from build123d import *

# Parameters (mm, degrees)
BOSS_EXTRU_1_DEPTH      = 10
BOSS_EXTRU_2_DEPTH      = 10
BOSS_EXTRU_2_DEPTH_BACK = 20
ESQUISSE2_W             = 69
ESQUISSE2_H             = 10
ESQUISSE3_W             = 50
ESQUISSE3_H             = 5
BOSS_EXTRU_3_DEPTH      = 15
CHANFREIN1_SIZE         = 5
ESQUISSE4_R             = 2.1
ENL_V_MAT_EXTRU_1_DEPTH = 15
ESQUISSE5_W             = 30
ESQUISSE5_H             = 5
BOSS_EXTRU_4_DEPTH      = 5
ESQUISSE6_W             = 50
ESQUISSE6_H             = 5
BOSS_EXTRU_5_DEPTH      = 15
CHANFREIN2_SIZE         = 5
ESQUISSE7_R             = 2.1
ENL_V_MAT_EXTRU_2_DEPTH = 15
ESQUISSE8_R             = 6
ENL_V_MAT_EXTRU_3_DEPTH = 20
CONG_1_R                = 5


with BuildPart() as part:
    # Esquisse1 → Boss.-Extru.1 (new body)
    with BuildSketch(Plane.XY):
        Polygon((0, 0), (0, 81), (-69, 81), (-69, 66), (-64, 66), (-64, 71), (-50, 71), (-50, 0), align=None)
    extrude(amount=BOSS_EXTRU_1_DEPTH)

    # Esquisse2 → Boss.-Extru.2 (add, two sides: drawn at the far end of the back side and taken through both)
    with BuildSketch(Plane.XY.offset(10).offset(-BOSS_EXTRU_2_DEPTH_BACK)):
        with Locations((-34.5, 76)):
            Rectangle(ESQUISSE2_W, ESQUISSE2_H)
    extrude(amount=BOSS_EXTRU_2_DEPTH + BOSS_EXTRU_2_DEPTH_BACK)

    # Esquisse3 → Boss.-Extru.3 (add)
    with BuildSketch(Plane(origin=(0, 0, 0), x_dir=(-1, 0, 0), z_dir=(0, 0, -1))):
        with Locations((25, 2.5)):
            Rectangle(ESQUISSE3_W, ESQUISSE3_H)
    extrude(amount=BOSS_EXTRU_3_DEPTH)

    # Chanfrein1
    chanfrein1_edges = [part.edges().sort_by_distance(p)[0] for p in [
        (-25, 5, 0),
    ]]
    chamfer(chanfrein1_edges, length=CHANFREIN1_SIZE)

    # Esquisse4 → Enlèv. mat.-Extru.1 (cut)
    with BuildSketch(Plane(origin=(0, 5, 0), x_dir=(1, 0, 0), z_dir=(0, 1, 0))):
        with Locations(Location((-40, 10, 0), (0, 0, 180))):
            Circle(ESQUISSE4_R)
        with Locations(Location((-10, 10, 0), (0, 0, 180))):
            Circle(ESQUISSE4_R)
    extrude(amount=-ENL_V_MAT_EXTRU_1_DEPTH, mode=Mode.SUBTRACT)

    # Esquisse5 → Boss.-Extru.4 (add)
    with BuildSketch(Plane.ZY.offset(69)):
        with Locations((5, 68.5)):
            Rectangle(ESQUISSE5_W, ESQUISSE5_H)
    extrude(amount=-BOSS_EXTRU_4_DEPTH)

    # Esquisse6 → Boss.-Extru.5 (add)
    with BuildSketch(Plane.XY.offset(10)):
        with Locations((-25, 13.5)):
            Rectangle(ESQUISSE6_W, ESQUISSE6_H)
    extrude(amount=BOSS_EXTRU_5_DEPTH)

    # Chanfrein2
    chanfrein2_edges = [part.edges().sort_by_distance(p)[0] for p in [
        (-25, 11, 10),
    ]]
    chamfer(chanfrein2_edges, length=CHANFREIN2_SIZE)

    # Esquisse7 → Enlèv. mat.-Extru.2 (cut)
    with BuildSketch(Plane.XZ.offset(-11)):
        with Locations((-10, 20)):
            Circle(ESQUISSE7_R)
        with Locations((-40, 20)):
            Circle(ESQUISSE7_R)
    extrude(amount=-ENL_V_MAT_EXTRU_2_DEPTH, mode=Mode.SUBTRACT)

    # Esquisse8 → Enlèv. mat.-Extru.3 (cut)
    with BuildSketch(Plane(origin=(0, 81, 0), x_dir=(1, 0, 0), z_dir=(0, 1, 0))):
        with Locations(Location((-35, 0, 0), (0, 0, 270))):
            Circle(ESQUISSE8_R)
    extrude(amount=-ENL_V_MAT_EXTRU_3_DEPTH, mode=Mode.SUBTRACT)

    # Congé1
    # the kernel refuses this fillet: 5 mm, written as the material it adds along each edge
    with BuildSketch(Plane(origin=(0, 10, 0), x_dir=(0, -0.7071067811865476, -0.7071067811865476), z_dir=(-1, 0, 0)), Plane(origin=(0, 5, -5), x_dir=(0, 0, -1), z_dir=(-1, 0, 0))) as cong_1_piece_1:
        with BuildLine():
            CenterArc((CONG_1_R * 0.414213562373, -CONG_1_R), CONG_1_R, 90, 45)
            Line((-CONG_1_R * 0.292893218813, -CONG_1_R * 0.292893218813), (0, 0))
            Line((0, 0), (CONG_1_R * 0.414213562373, 0))
        make_face()
    extrude(amount=50)
    # the kernel refuses this fillet: 5 mm, written as the material it takes off along each edge
    with BuildSketch(Plane(origin=(-81.5, 81, 20), x_dir=(0, -1, 0), z_dir=(1, 0, 0))) as cong_1_2_piece_1:
        with BuildLine():
            CenterArc((CONG_1_R, CONG_1_R), CONG_1_R, 180, 90)
            Line((0, CONG_1_R), (0, 0))
            Line((0, 0), (CONG_1_R, 0))
        make_face()
    extrude(amount=94, mode=Mode.SUBTRACT)
    with BuildSketch(Plane(origin=(12.5, 71, 20), x_dir=(0, 0, -1), z_dir=(-1, 0, 0))) as cong_1_2_piece_2:
        with BuildLine():
            CenterArc((CONG_1_R, -CONG_1_R), CONG_1_R, 90, 90)
            Line((0, -CONG_1_R), (0, 0))
            Line((0, 0), (CONG_1_R, 0))
        make_face()
    extrude(amount=76.5, mode=Mode.SUBTRACT)
    with BuildSketch(Plane(origin=(0, 71, -2.5), x_dir=(0, 1, 0), z_dir=(0, 0, 1))) as cong_1_2_piece_3_section:
        with BuildLine():
            CenterArc((CONG_1_R, CONG_1_R), CONG_1_R, 180, 90)
            Line((0, CONG_1_R), (0, 0))
            Line((0, 0), (CONG_1_R, 0))
        make_face()
    cong_1_2_piece_3 = extrude(amount=35, mode=Mode.PRIVATE)
    cong_1_2_piece_3 = split(cong_1_2_piece_3, bisect_by=Plane(origin=(-1.116839695, 72.116839695, 0), z_dir=(0, 0, -1)), keep=Keep.TOP, mode=Mode.PRIVATE)
    add(cong_1_2_piece_3, mode=Mode.SUBTRACT)
    with BuildSketch(Plane(origin=(0, 71, 10), x_dir=(0, 1, 0), z_dir=(0, 0, 1)), Plane(origin=(0, 71, -22.5), x_dir=(0, 1, 0), z_dir=(0, 0, 1))) as cong_1_2_piece_4:
        with BuildLine():
            CenterArc((CONG_1_R, CONG_1_R), CONG_1_R, 180, 90)
            Line((0, CONG_1_R), (0, 0))
            Line((0, 0), (CONG_1_R, 0))
        make_face()
    extrude(amount=22.5, mode=Mode.SUBTRACT)
    with BuildSketch(Plane(origin=(0, 71, -22.5), x_dir=(0, 1, 0), z_dir=(0, 0, 1))) as cong_1_2_piece_5_section:
        with BuildLine():
            CenterArc((CONG_1_R, CONG_1_R), CONG_1_R, 180, 90)
            Line((0, CONG_1_R), (0, 0))
            Line((0, 0), (CONG_1_R, 0))
        make_face()
    cong_1_2_piece_5 = extrude(amount=35, mode=Mode.PRIVATE)
    cong_1_2_piece_5 = split(cong_1_2_piece_5, bisect_by=Plane(origin=(-1.116839695, 72.116839695, 10), z_dir=(0, 0, 1)), keep=Keep.TOP, mode=Mode.PRIVATE)
    add(cong_1_2_piece_5, mode=Mode.SUBTRACT)
    with BuildSketch(Plane(origin=(0, 81, -22.5), x_dir=(0, -1, 0), z_dir=(0, 0, 1)), Plane(origin=(-69, 81, -22.5), x_dir=(1, 0, 0), z_dir=(0, 0, 1))) as cong_1_2_piece_6:
        with BuildLine():
            CenterArc((CONG_1_R, -CONG_1_R), CONG_1_R, 90, 90)
            Line((0, -CONG_1_R), (0, 0))
            Line((0, 0), (CONG_1_R, 0))
        make_face()
    extrude(amount=55, mode=Mode.SUBTRACT)
    with BuildSketch(Plane(origin=(12.5, 71, -10), x_dir=(0, 0, 1), z_dir=(-1, 0, 0))) as cong_1_2_piece_7:
        with BuildLine():
            CenterArc((CONG_1_R, CONG_1_R), CONG_1_R, 180, 90)
            Line((0, CONG_1_R), (0, 0))
            Line((0, 0), (CONG_1_R, 0))
        make_face()
    extrude(amount=76.5, mode=Mode.SUBTRACT)
    with BuildSketch(Plane(origin=(-81.5, 81, -10), x_dir=(0, -1, 0), z_dir=(1, 0, 0))) as cong_1_2_piece_8:
        with BuildLine():
            CenterArc((CONG_1_R, -CONG_1_R), CONG_1_R, 90, 90)
            Line((0, -CONG_1_R), (0, 0))
            Line((0, 0), (CONG_1_R, 0))
        make_face()
    extrude(amount=94, mode=Mode.SUBTRACT)
    with BuildSketch(Plane(origin=(-69, 66, -22.5), x_dir=(1, 0, 0), z_dir=(0, 0, 1))) as cong_1_2_piece_9:
        with BuildLine():
            CenterArc((CONG_1_R, CONG_1_R), CONG_1_R, 180, 90)
            Line((0, CONG_1_R), (0, 0))
            Line((0, 0), (CONG_1_R, 0))
        make_face()
    extrude(amount=55, mode=Mode.SUBTRACT)


solid = part.part
Here's how the part is built. I have some questions about the finished solid (model axes, mm). A direction names the side the tool comes from. Coordinates: 2 decimals unless noted, no trailing zeros. Write each loop counter-clockwise with the first axis right and the second up, starting at its lowest first coordinate (ties: lowest second). Pieces come first, ordered by that corner, then holes.
Item 1: If I drill on line 1 (Z direction, x = -40, y = 2); line 2 (Z direction, x = -10, y = 14); line 3 (Z direction, x = -27.5, y = 69), over which ranges is the centre line in solid material (lowest first)?
Item 2: If we mould it in two halves opening along Y, with no side actions, what happens to faces 6 (the flat face through (-35, 81, 7)), 7 (the flat face through (-50, 31, 6)), 8 (the flat face through (-25, 9, 13)), 9 (the flat face through (-25, 46, 10))? For each: +Y half, -Y half, draft (parallel to the pull), parting line (faces both ways), or undercut.
Item 3: I want a section at A-A on x = -10. Write out the boundary of the cut face in (y, z), and give its area (3 significant figures).
Item 4: Will these pins go through, and if not, where does the flat tip stop? pin 1 (2.5 mm diameter, centred on x = -66, y = 69.5, fed in from +Z); pin 2 (2.5 mm diameter, centred on x = -10, z = -10, fed in from -Y); pin 3 (2.5 mm diameter, centred on x = -17, z = -2, fed in from -Y); pin 4 (5.5 mm diameter, centred on x = -66.5, y = 73, fed in from -Z).
Item 5: I want a section at C-C on y = 72.5. Write out the boundary of the cut face in (x, z).
Item 6: I want a section at B-B on x = -35. Write out the boundary of the cut face in (y, z).
Item 7: I want a section at D-D on z = 19. Write out the boundary of the cut face in (x, y), and give its area (3 significant figures).
Item 8: On a 3-axis mill with a long thin cutter (end or side, diameter ignored), from which of +Z, -Z, +X, -X, +Y, -Y can I reach the whole of each face in a straight line? I mean faces 1 (the flat face through (-25, 3, 10)), 2 (the cylindrical face through (-38.452, 2.535, -8.581)), 3 (the cylindrical face through (-24.65, 10.13, -0.39)), 4 (the flat face through (-25, 3, -15)), 5 (the flat face through (-25, 14, 25)). Say none if no direction works.
Findings below:
1. line 1: z = -15 to -12.1, -7.9 to 10
1. line 2: z = 0 to 17.9, 22.1 to 25
1. line 3: z = 0 to 10
2. face 6: +Y half
2. face 7: draft
2. face 8: -Y half
2. face 9: undercut
3. outline: (0, -15) - (5, -15) - (5, -12.1) - (0, -12.1) - close; (0, -7.9) - (5, -7.9) - (5, -7.07) arc R5 cw to (6.46, -3.54) - (8.54, -1.46) arc R5 cw to (12.07, 0) - (71, 0) - (71, -5) arc R5 ccw to (81, -5) - (81, 15) arc R5 ccw to (71, 15) - (71, 10) - (16, 10) - (16, 17.9) - (11, 17.9) - (11, 15) - (6, 10) - (0, 10) - close; (11, 22.1) - (16, 22.1) - (16, 25) - (11, 25) - close
3. area: 1,120 mm2
4. pin 1: stops at z = 20
4. pin 2: stops at y = 72.69
4. pin 3: stops at y = 0
4. pin 4: stops at z = -10
5. outline: (-69, -10) - (-64, -10) - (-64, -8.57) - (-1.43, -8.57) - (-1.43, 0) - (0, 0) - (0, 10) - (-1.43, 10) - (-1.43, 18.57) - (-64, 18.57) - (-64, 20) - (-69, 20) - close; hole circle Ø12 at (-35, 0)
6. outline: (0, -15) - (5, -15) - (5, -7.07) arc R5 cw to (6.46, -3.54) - (8.54, -1.46) arc R5 cw to (12.07, 0) - (61, 0) - (61, 6) - (81, 6) - (81, 15) arc R5 ccw to (71, 15) - (71, 10) - (16, 10) - (16, 25) - (11, 25) - (11, 15) - (6, 10) - (0, 10) - close; (71.1, -6) arc R5 ccw to (80.9, -6) - close
7. outline: (-69, 71) arc R5 ccw to (-64, 66) - (-64, 73) - (-1, 73) arc R5 ccw to (-1, 79) - (-68, 79) arc R5 ccw to (-69, 76) - close; (-50, 11) - (-41.85, 11) - (-41.85, 16) - (-50, 16) - close; (-38.15, 11) - (-11.85, 11) - (-11.85, 16) - (-38.15, 16) - close; (-8.15, 11) - (0, 11) - (0, 16) - (-8.15, 16) - close
7. area: 654 mm2
8. face 1: +Z, +X, -X, -Y
8. face 2: -Y
8. face 3: -Z, +X, -X
8. face 4: -Z, +X, -X, +Y, -Y
8. face 5: +Z, +X, -X, +Y, -Y
